Geometry: final body of the model. Coordinates: model frame, mm. A direction names the side the tool comes from. Coordinates: 2 decimals unless noted, no trailing zeros. Write each loop counter-clockwise with the first axis right and the second up, starting at its lowest first coordinate (ties: lowest second). Pieces come first, ordered by that corner, then holes. Notation, with made-up numbers: (82.25, 63) - (141.25, 63) arc R27 ccw to (141.25, 83) - close; hole circle Ø10 at (2.5, 38). An arc over 180 degrees is marked (long way). Answer as a JSON object with one key per item and string values. Group by question number.
Item 1: Mould query, pull axis Z, two halves, no side actions, for faces 1 (the conical face through (-10.676, -48.079, -0.563)), 2 (the flat face through (11, 1, -2.5)), 3 (the cylindrical face through (-7.03, -7.11, 0.04)). Classes: pulls with the +Z half, pulls with the -Z half, needs draft (parallel to the pull), parting line crosses it, or undercut.
Item 2: Line query: line 1 along Y through (x, z) = (0, -8.5); line 2 along Z through (x, y) = (-36, -24); line 3 along Y through (x, z) = (-34.5, -1.75). Output: solid intervals per line, ascending. Write a range as from..to.
Item 3: Section B-B on x = -12. State how many separate pieces and enclosed holes the cut face has, and give its area (3 significant figures).
Item 4: Set-up query: faces 4 (the cylindrical face through (26.34, 41.32, -0.01)), 5 (the flat face through (20, 0.5, 5)), 6 (the flat face through (5.027, 25, 0)), 7 (the flat face through (-1.3, 0, -17.5)), 8 (the flat face through (17.5, 4, 6)). Return all of +Z, -Z, +X, -X, +Y, -Y with unobstructed straight access to the full face (end or side cutting, diameter ignored); none if empty.
Item 5: Section A-A on z = -11.5. Return loops of the section in (x, y).
Item 6: First-contact query: pin 1 Ø2.5 at (y, z) = (-23, 1) entering from +X; pin 2 Ø8 at (x, z) = (38.5, -1) entering from -Y; pin 3 Ø5.5 at (y, z) = (25.5, -1) entering from +X; pin 4 Ø3.5 at (x, y) = (0, 0) entering from -Z. Flat tips, straight axial feed; report the tip coordinate or a pass-through.
```python
from build123d import *

# Parameters (mm, degrees)
CUT_EXTRUDE2_REACH      = 7
SKETCH6_W               = 5
SKETCH6_H               = 4.5
BOSS_EXTRUDE1_DEPTH     = 6
SKETCH7_W               = 5
SKETCH7_H               = 3
BOSS_EXTRUDE2_DEPTH     = 5
SKETCH23_R              = 3
BOSS_EXTRUDE5_DEPTH     = 15
SKETCH5_R               = 1.1
CUT_EXTRUDE3_DEPTH      = 7
CUT_EXTRUDE3_DEPTH_BACK = 21
SKETCH22_R              = 2.5
CUT_EXTRUDE4_DEPTH      = 9.5
CUT_EXTRUDE4_DEPTH_BACK = 18.5
SKETCH21_R              = 0.25
CUT_EXTRUDE5_DEPTH      = 2.5


with BuildPart() as part:
    # Sketch2 → Revolve1 (revolve)
    with BuildSketch(Plane(origin=(0, 0, 0), x_dir=(1, 0, 0), z_dir=(0, 1, 0))):
        Polygon((53, -1.5), (49, -0.5), (49, 0.5), (53, 1.5), (53, 2.5), (50, 2.5), (0, 2.5), (0, -2.5), (50, -2.5), (53, -2.5), align=None)
    revolve(axis=Axis((0, 0, -2.5), (0, 0, 1)))

    # Sketch4 → Cut-Extrude2 (cut, up to next)
    with BuildSketch(Plane.XY.offset(2.5), mode=Mode.PRIVATE) as cut_extrude2_sk1:
        with BuildLine():
            Line((5.026990014, 8.644615168), (5.026990014, 42.705144554))
            ThreePointArc((5.026990014, 42.705144554), (30.415198012, 30.395982134), (42.708313008, 5))
            Line((42.708313008, 5), (8.660254038, 5))
            ThreePointArc((8.660254038, 5), (7.082087783, 7.06003064), (5.026990014, 8.644615168))
        make_face()
    cut_extrude2_tool1 = extrude(cut_extrude2_sk1.sketch, amount=-CUT_EXTRUDE2_REACH, mode=Mode.PRIVATE) & part.part
    add(cut_extrude2_tool1.solids().sort_by_distance((20.56337, 20.545095, 2.5))[0], mode=Mode.SUBTRACT)
    # Sketch4 → Cut-Extrude2 (cut, up to next)
    with BuildSketch(Plane.XY.offset(2.5), mode=Mode.PRIVATE) as cut_extrude2_sk2:
        with BuildLine():
            Line((-4.973009986, -42.711464172), (-4.973009986, -8.675780754))
            ThreePointArc((-4.973009986, -8.675780754), (-7.060050497, -7.082067988), (-8.660254038, -5))
            Line((-8.660254038, -5), (-42.708313008, -5))
            ThreePointArc((-42.708313008, -5), (-30.395982845, -30.415197302), (-4.973009986, -42.711464172))
        make_face()
    cut_extrude2_tool2 = extrude(cut_extrude2_sk2.sketch, amount=-CUT_EXTRUDE2_REACH, mode=Mode.PRIVATE) & part.part
    add(cut_extrude2_tool2.solids().sort_by_distance((-20.535898, -20.554166, 2.5))[0], mode=Mode.SUBTRACT)
    # Sketch4 → Cut-Extrude2 (cut, up to next)
    with BuildSketch(Plane.XY.offset(2.5), mode=Mode.PRIVATE) as cut_extrude2_sk3:
        with BuildLine():
            Line((5.026990014, -42.705144554), (5.026990014, -8.644615168))
            ThreePointArc((5.026990014, -8.644615168), (7.082087783, -7.06003064), (8.660254038, -5))
            Line((8.660254038, -5), (42.708313008, -5))
            ThreePointArc((42.708313008, -5), (30.415198012, -30.395982134), (5.026990014, -42.705144554))
        make_face()
    cut_extrude2_tool3 = extrude(cut_extrude2_sk3.sketch, amount=-CUT_EXTRUDE2_REACH, mode=Mode.PRIVATE) & part.part
    add(cut_extrude2_tool3.solids().sort_by_distance((20.56337, -20.545095, 2.5))[0], mode=Mode.SUBTRACT)
    # Sketch4 → Cut-Extrude2 (cut, up to next)
    with BuildSketch(Plane.XY.offset(2.5), mode=Mode.PRIVATE) as cut_extrude2_sk4:
        with BuildLine():
            Line((-42.708313008, 5), (-8.660254038, 5))
            ThreePointArc((-8.660254038, 5), (-7.060050497, 7.082067988), (-4.973009986, 8.675780754))
            Line((-4.973009986, 8.675780754), (-4.973009986, 42.711464172))
            ThreePointArc((-4.973009986, 42.711464172), (-30.395982845, 30.415197302), (-42.708313008, 5))
        make_face()
    cut_extrude2_tool4 = extrude(cut_extrude2_sk4.sketch, amount=-CUT_EXTRUDE2_REACH, mode=Mode.PRIVATE) & part.part
    add(cut_extrude2_tool4.solids().sort_by_distance((-20.535898, 20.554166, 2.5))[0], mode=Mode.SUBTRACT)

    # Sketch6 → Boss-Extrude1 (add)
    with BuildSketch(Plane.XY.offset(2.5)):
        with Locations((20, 2.75)):
            Rectangle(SKETCH6_W, SKETCH6_H)
    extrude(amount=BOSS_EXTRUDE1_DEPTH)

    # Sketch7 → Boss-Extrude2 (add)
    with BuildSketch(Plane(origin=(0, 5, 0), x_dir=(1, 0, 0), z_dir=(0, 1, 0))):
        with Locations((20, -7)):
            Rectangle(SKETCH7_W, SKETCH7_H)
    extrude(amount=BOSS_EXTRUDE2_DEPTH)

    # Sketch23 → Boss-Extrude5 (add)
    with BuildSketch(Plane(origin=(0, 0, -2.5), x_dir=(-1, 0, 0), z_dir=(0, 0, -1))):
        Circle(SKETCH23_R)
    extrude(amount=BOSS_EXTRUDE5_DEPTH)

    # Sketch5 → Cut-Extrude3 (cut, two sides)
    with BuildSketch(Plane.XY.offset(2.5)) as cut_extrude3_sk:
        Circle(SKETCH5_R)
    extrude(amount=CUT_EXTRUDE3_DEPTH, mode=Mode.SUBTRACT)
    extrude(cut_extrude3_sk.sketch, amount=-CUT_EXTRUDE3_DEPTH_BACK, mode=Mode.SUBTRACT)

    # Sketch22 → Cut-Extrude4 (cut, two sides)
    with BuildSketch(Plane.XY) as cut_extrude4_sk:
        with Locations((53, 0)):
            Circle(SKETCH22_R)
    extrude(amount=CUT_EXTRUDE4_DEPTH, mode=Mode.SUBTRACT)
    extrude(cut_extrude4_sk.sketch, amount=-CUT_EXTRUDE4_DEPTH_BACK, mode=Mode.SUBTRACT)

    # Sketch21 → Cut-Extrude5 (cut)
    with BuildSketch(Plane(origin=(49, 0, 0), x_dir=(0, 0, -1), z_dir=(1, 0, 0))):
        Circle(SKETCH21_R)
    extrude(amount=-CUT_EXTRUDE5_DEPTH, mode=Mode.SUBTRACT)


solid = part.part
```
Checks:
{
 "1": {"face 1": "undercut", "face 2": "pulls with the -Z half", "face 3": "needs draft"},
 "2": {"line 1": "-3..-1.1, 1.1..3", "line 2": "-2.5..2.5", "line 3": "-40.23..-25.67, -5..5, 25.67..40.23"},
 "3": {"separate pieces": "3", "enclosed holes": "0", "area": "137 mm^2"},
 "4": {"face 4": "none", "face 5": "+Z, +X, -X, -Y", "face 6": "+Z, -Z", "face 7": "-Z, +X, -X, +Y, -Y", "face 8": "+Z, -X, +Y, -Y"},
 "5": {"outline": "circle Ø6 at (0, 0); hole circle Ø2.2 at (0, 0)"},
 "6": {"pin 1": "x = 48.28", "pin 2": "y = -40.21", "pin 3": "x = 47.85", "pin 4": "z = -17.5"}
}
